Here's how the part is built. I have some questions about the finished solid (model axes, mm). Face numbers are marked on the shaded views. A direction names the side the tool comes from. Give positions to 0.01 mm unless a question says otherwise; leave off trailing zeros. Loops run counter-clockwise (first coordinate to the right, second up) from the corner with the lowest first, then second, coordinate; pieces in that order, holes last. Notation, with made-up numbers: (67.5, 4) - (81.5, 4) arc R28 ccw to (81.5, 33) - close; hole circle Ø6 at (-24.5, 23). An arc over 180 degrees is marked (long way). Use one line per item in the form item = value.
from build123d import *

# Parameters (mm, degrees)
EXTRUDE001_DEPTH = 45
EXTRUDE_DEPTH    = 5
FACE005_R        = 2.5
EXTRUDE005_DEPTH = 5
SKETCH004_R      = 2.5
EXTRUDE004_DEPTH = 5
FACE003_R        = 2.5
EXTRUDE003_DEPTH = 5
EXTRUDE002_DEPTH = 20
FILLET_R         = 5
FILLET001_R      = 5
FILLET002_R      = 5
FILLET003_R      = 5
FILLET004_R      = 1.5
FILLET005_R      = 1.5
FILLET006_R      = 1.5
FILLET007_R      = 1.5


with BuildPart() as extrude001:
    # Face001 → Extrude001 (new body)
    with BuildSketch(Plane(origin=(7.142857, 100, 5), x_dir=(0, 1, 0), z_dir=(0, 0, 1))):
        Polygon((-120, -12.857143), (-120, -17.857143), (-95, -17.857143), (-95, 2.142857), (95, 2.142857), (95, -17.857143), (120, -17.857143), (120, -12.857143), (100, -12.857143), (100, 7.142857), (-100, 7.142857), (-100, -12.857143), align=None)
    extrude(amount=EXTRUDE001_DEPTH)


with BuildPart() as fusion:
    # Sketch → Extrude (new body)
    with BuildSketch(Plane.XY):
        Polygon((20, -20), (20, 0), (0, 0), (0, 200), (20, 200), (20, 220), (25, 220), (25, -20), align=None)
    extrude(amount=EXTRUDE_DEPTH)

    # Fusion: union Extrude001
    add(extrude001.part)


with BuildPart() as extrude005:
    # Face005 → Extrude005 (new body)
    with BuildSketch(Plane(origin=(10, 5, 60), x_dir=(1, 0, 0), z_dir=(0, 1, 0))):
        Circle(FACE005_R)
    extrude(amount=-EXTRUDE005_DEPTH)


with BuildPart() as extrude004:
    # Sketch004 (on Face12 of Cut) → Extrude004 (new body)
    with BuildSketch(Plane.XZ.offset(-195)):
        with Locations((10, 60)):
            Circle(SKETCH004_R)
    extrude(amount=-EXTRUDE004_DEPTH)


with BuildPart() as extrude003:
    # Face003 → Extrude003 (new body)
    with BuildSketch(Plane(origin=(25, -10, 60), x_dir=(0, -1, 0), z_dir=(1, 0, 0))):
        Circle(FACE003_R)
        with Locations((-220, 0)):
            Circle(FACE003_R)
    extrude(amount=-EXTRUDE003_DEPTH)


with BuildPart() as fillet007:
    # Face002 → Extrude002 (new body)
    with BuildSketch(Plane(origin=(16.944444, -3.055556, 50), x_dir=(0, 1, 0), z_dir=(0, 0, 1))):
        Polygon((8.055556, -8.055556), (8.055556, 16.944444), (3.055556, 16.944444), (3.055556, -3.055556), (-16.944444, -3.055556), (-16.944444, -8.055556), align=None)
        Polygon((203.055556, 16.944444), (198.055556, 16.944444), (198.055556, -8.055556), (223.055556, -8.055556), (223.055556, -3.055556), (203.055556, -3.055556), align=None)
    extrude(amount=EXTRUDE002_DEPTH)

    # Cut: cut Extrude003
    add(extrude003.part, mode=Mode.SUBTRACT)

    # Cut001: cut Extrude004
    add(extrude004.part, mode=Mode.SUBTRACT)

    # Cut002: cut Extrude005
    add(extrude005.part, mode=Mode.SUBTRACT)

    # Fusion001: union Fusion
    add(fusion.part)

    # Fillet
    fillet_edges = [fillet007.edges().sort_by_distance(p)[0] for p in [
        (22.5, 220, 70),
    ]]
    fillet(fillet_edges, radius=FILLET_R)

    # Fillet001
    fillet001_edges = [fillet007.edges().sort_by_distance(p)[0] for p in [
        (0, 197.5, 70),
    ]]
    fillet(fillet001_edges, radius=FILLET001_R)

    # Fillet002
    fillet002_edges = [fillet007.edges().sort_by_distance(p)[0] for p in [
        (22.5, -20, 70),
    ]]
    fillet(fillet002_edges, radius=FILLET002_R)

    # Fillet003
    fillet003_edges = [fillet007.edges().sort_by_distance(p)[0] for p in [
        (0, 2.5, 70),
    ]]
    fillet(fillet003_edges, radius=FILLET003_R)

    # Fillet004
    fillet004_edges = [fillet007.edges().sort_by_distance(p)[0] for p in [
        (5, 100, 50),
    ]]
    fillet(fillet004_edges, radius=FILLET004_R)

    # Fillet005
    fillet005_edges = [fillet007.edges().sort_by_distance(p)[0] for p in [
        (0, 100, 50),
    ]]
    fillet(fillet005_edges, radius=FILLET005_R)

    # Fillet006
    fillet006_edges = [fillet007.edges().sort_by_distance(p)[0] for p in [
        (0, 195, 57.5),
        (1.464466, 195, 68.535534),
        (15, 195, 70),
    ]]
    fillet(fillet006_edges, radius=FILLET006_R)

    # Fillet007
    fillet007_edges = [fillet007.edges().sort_by_distance(p)[0] for p in [
        (0, 5, 57.5),
    ]]
    fillet(fillet007_edges, radius=FILLET007_R)


solid = fillet007.part
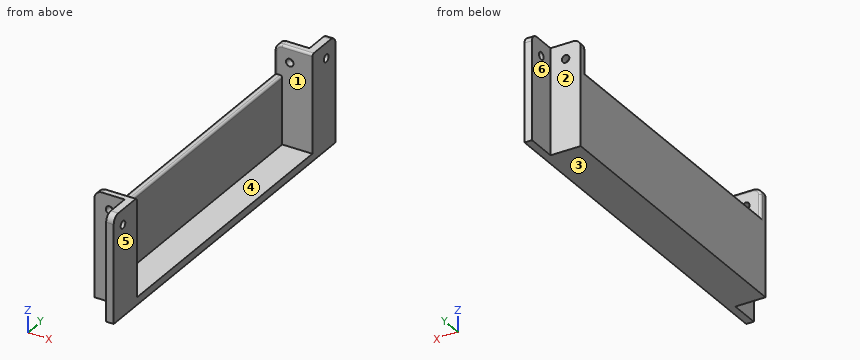
(1) If we section it at B-B (y = -10): List the corners of the cut face in (x, z) for me.
Geometry says:
outline = (20, 0) - (25, 0) - (25, 57.5) - (20, 57.5) - close; (20, 62.5) - (25, 62.5) - (25, 70) - (20, 70) - close
(2) If we section it at C-C (z = 60): Give the number of separate pieces and of enclosed holes in the cut face, plus the area to 3 significant figures.
Geometry says:
separate_pieces = 6
enclosed_holes = 0
area = 349 mm²
(3) If we section it at A-A (x = 10): List the corners of the cut face in (y, z) for me.
Geometry says:
outline = (0, 0) - (200, 0) - (200, 57.5) - (195, 57.5) - (195, 5) - (5, 5) - (5, 57.5) - (0, 57.5) - close; (0, 62.5) - (5, 62.5) - (5, 68.5) arc R1.5 ccw to (3.5, 70) - (0, 70) - close; (195, 62.5) - (200, 62.5) - (200, 70) - (196.5, 70) arc R1.5 ccw to (195, 68.5) - close
(4) For P1, Ø6, axis at y = -10, z = 60, coming from the -X side; P2, Ø4, axis at y = 34, z = 35.5, coming from the +X side; P3, Ø10, axis at x = 15.5, y = 75.5, coming from the +Z side, each with a flat end and sliding along its axis, tell me the tip position at first contact or that it passes through.
Geometry says:
P1 = 20
P2 = 5
P3 = 5
(5) If I drill on probe 1 along Y at (x, z) = (21.25, 60); probe 2 along Y at (x, z) = (24.25, 28.5); probe 3 along Y at (x, z) = (17.25, 52.5), over which ranges is the centre line in solid material (lowest first)?
Geometry says:
probe_1 = -20 to -12.5, -7.5 to 5, 195 to 207.5, 212.5 to 220
probe_2 = -20 to 5, 195 to 220
probe_3 = 0 to 5, 195 to 200
(6) For the marked faces 4, 5 and 6, which set-ups out of +Z, -Z, +X, -X, +Y, -Y let a thin tool reach every point of the face, with its end or its side?
Geometry says:
face_4 = +Z, +X
face_5 = +Z, -Z, +X, +Y, -Y
face_6 = +Z, -Z, -X, +Y
(7) Thinking about a two-plate mould opening in Y: for the marked faces 1, 2 and 3, which applies, pulls with the +Y half, pulls with the -Y half, needs draft (parallel to the pull), parting line crosses it, or undercut?
Geometry says:
face_1 = undercut
face_2 = pulls with the +Y half
face_3 = needs draft
(8) If we section it at D-D (y = 150): List the corners of the cut face in (x, z) for me, plus the area to 3 significant figures.
Geometry says:
outline = (0, 0) - (25, 0) - (25, 5) - (5, 5) - (5, 48.5) arc R1.5 ccw to (3.5, 50) - (1.5, 50) arc R1.5 ccw to (0, 48.5) - close
area = 349 mm²
